The drawing under review shows one solid part. Ordinate dimensions are in mm from its lowest x, y, z. Coordinates: 2 decimals unless noted, no trailing zeros. Loops run counter-clockwise (first coordinate to the right, second up) from the corner with the lowest first, then second, coordinate; pieces in that order, holes last. Notation, with made-up numbers: (47.5, -17.5) -> (67.5, -17.5) arc R30 ccw to (67.5, 9.5) -> close; hole circle Ø10 at (80.25, 85.5). An arc over 180 degrees is marked (long way). Use a Markdown table: item, result.
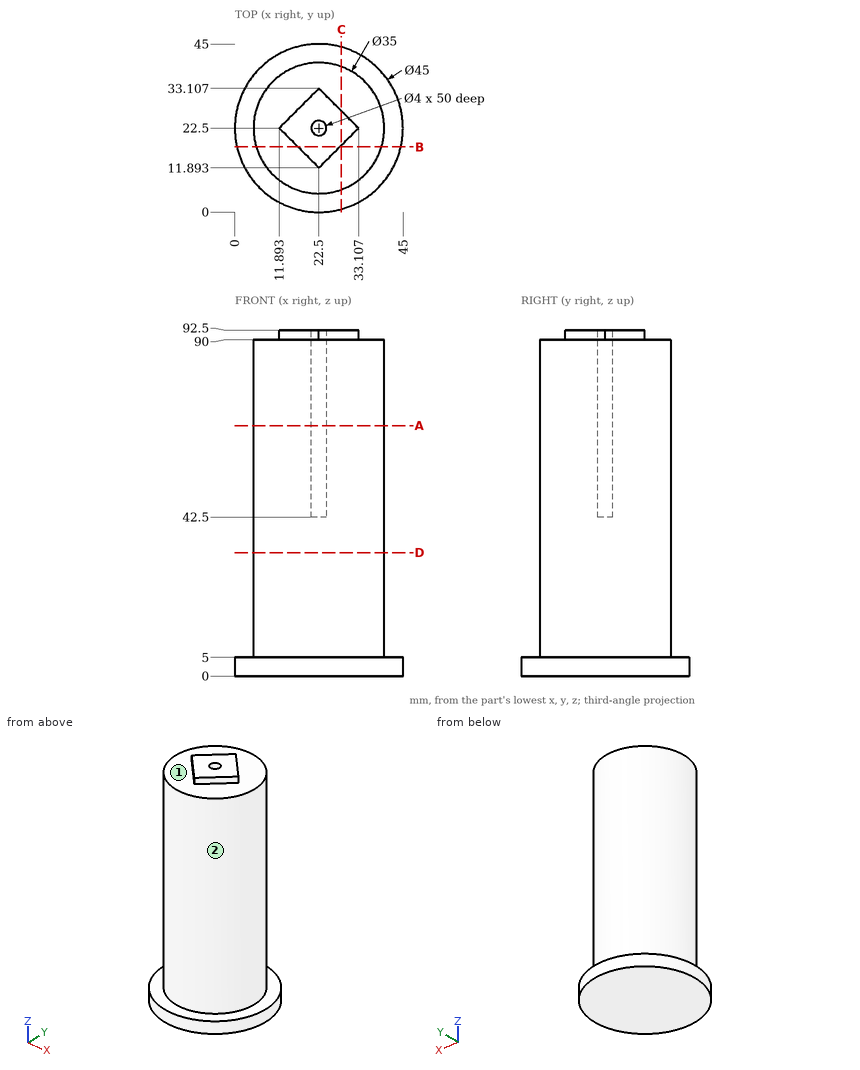
(1) For pin 1 Ø6 at (y, z) = (31, 22) entering from -X; pin 2 Ø1.5 at (x, y) = (38, 30.5) entering from +Z; pin 3 Ø12 at (x, z) = (34.5, 74) entering from -Y, all flat-tipped, find the tip position at first contact; note any pin that passes through.
Found:
| item | result |
|---|---|
| pin 1 | stops at x = 5.89 |
| pin 2 | stops at z = 90 |
| pin 3 | stops at y = 6.06 |
(2) Mouldability with a two-part tool opening along Y and no side actions: class the marked faces 1 and 2 as pulls with the +Y half, pulls with the -Y half, needs draft (parallel to the pull), parting line crosses it, or undercut.
Found:
| item | result |
|---|---|
| face 1 | needs draft |
| face 2 | parting line crosses it |
(3) Take a section at C-C on x = 28.5. Write out the cut boundary in (y, z) (1 decimal).
Found:
| item | result |
|---|---|
| outline | (0.8, 0) -> (44.2, 0) -> (44.2, 5) -> (38.9, 5) -> (38.9, 90) -> (27.1, 90) -> (27.1, 92.5) -> (17.9, 92.5) -> (17.9, 90) -> (6.1, 90) -> (6.1, 5) -> (0.8, 5) -> close |
(4) Take a section at A-A on z = 67. Write out the cut boundary in (x, y).
Found:
| item | result |
|---|---|
| outline | circle Ø35 at (22.5, 22.5); hole circle Ø4 at (22.5, 22.5) |
(5) Take a section at D-D on z = 33. Write out the cut boundary in (x, y).
Found:
| item | result |
|---|---|
| outline | circle Ø35 at (22.5, 22.5) |
(6) For line 1 along Y through (x, z) = (22.5, 58); line 2 along Z through (x, y) = (6.5, 38); line 3 along Z through (x, y) = (25, 35), list the stretches that pass through material, from the lowest coordinate up.
Found:
| item | result |
|---|---|
| line 1 | y = 5 to 20.5, 24.5 to 40 |
| line 2 | z = 0 to 5 |
| line 3 | z = 0 to 90 |
(7) Take a section at B-B on y = 17.5. Write out the cut boundary in (x, z), plus the area to 3 significant figures.
Found:
| item | result |
|---|---|
| outline | (0.56, 0) -> (44.44, 0) -> (44.44, 5) -> (39.27, 5) -> (39.27, 90) -> (28.11, 90) -> (28.11, 92.5) -> (16.89, 92.5) -> (16.89, 90) -> (5.73, 90) -> (5.73, 5) -> (0.56, 5) -> close |
| area | 3,100 mm^2 |
